Here's how the part is built. I have some questions about the finished solid (model axes, mm). A direction names the side the tool comes from. Coordinates: 2 decimals unless noted, no trailing zeros. Write each loop counter-clockwise with the first axis right and the second up, starting at its lowest first coordinate (ties: lowest second). Pieces come first, ordered by that corner, then holes.
from build123d import *

# Parameters (mm, degrees)
ESQUISSE1_W                     = 50
ESQUISSE1_H                     = 45
MAIN_EXTRUSION_DEPTH            = 20
ESQUISSE5_R                     = 8
GEAR_LINEAR_HOLES_DEPTH         = 21
FIXING_EXTRUSION_DEPTH          = 25
ESQUISSE13_W                    = 50
ESQUISSE13_H                    = 7.2
ROLLINGBALLHORIZONTALHOLE_DEPTH = 11
FRONTHOLE_DEPTH                 = 22
ESQUISSE15_R                    = 1.6
BOTTOMFIXINGHOLE_DEPTH          = 36.1
ESQUISSE12_R                    = 16
REDUCTORMAINHOLE_DEPTH          = 5
REDUCTORFRONTFIXINGHOLE_DEPTH   = 3
ESQUISSE17_R                    = 1.6
MOTORFIXINGHOLE_DEPTH           = 31.1
ESQUISSE19_R                    = 3
ENL_V_MAT_EXTRU_5_DEPTH         = 3
SKETCH2_W                       = 1.5
SKETCH2_H                       = 11
CUTFORMAKERBEAMPROFILE_DEPTH    = 51
CUTFORDISTRIBUTORGRABBER_DEPTH  = 21
SKETCH4_R                       = 1.3
HOLETOBLOCKBEHIND_DEPTH         = 12


with BuildPart() as part:
    # Esquisse1 → Main Extrusion (new body)
    with BuildSketch(Plane.XY):
        Rectangle(ESQUISSE1_W, ESQUISSE1_H)
    extrude(amount=MAIN_EXTRUSION_DEPTH)

    # Esquisse5 → Gear Linear Holes (cut, through all)
    with BuildSketch(Plane.XY.offset(20)):
        with Locations((-7, 2.5)):
            Circle(ESQUISSE5_R)
    extrude(amount=-GEAR_LINEAR_HOLES_DEPTH, mode=Mode.SUBTRACT)

    # Esquisse8 → Fixing Extrusion (add, symmetric)
    with BuildSketch(Plane(origin=(0, 0, 0), x_dir=(0, 0, -1), z_dir=(1, 0, 0))):
        Polygon((-20, -25.5), (-20, -29.05), (-21, -29.05), (-21, -31.95), (-20, -31.95), (-20, -35.5), (0, -35.5), (0, -21.5), (-35.1, -21.5), (-35.1, -35.5), (-30.1, -35.5), (-30.1, -31.95), (-29.1, -31.95), (-29.1, -29.05), (-30.1, -29.05), (-30.1, -25.5), (-26.5, -25.5), (-26.5, -26.5), (-23.6, -26.5), (-23.6, -25.5), align=None)
    extrude(amount=FIXING_EXTRUSION_DEPTH, both=True)

    # Esquisse13 → RollingBallHorizontalHole (cut)
    with BuildSketch(Plane.XY.offset(20)):
        with Locations((0, -14.4)):
            Rectangle(ESQUISSE13_W, ESQUISSE13_H)
    extrude(amount=-ROLLINGBALLHORIZONTALHOLE_DEPTH, mode=Mode.SUBTRACT)

    # Esquisse14 → FrontHole (cut)
    with BuildSketch(Plane.ZY.offset(25)):
        Polygon((0, -23), (20, -23), (20, -18), (35.1, -18), (35.1, -35.5), (0, -35.5), align=None)
    extrude(amount=-FRONTHOLE_DEPTH, mode=Mode.SUBTRACT)

    # Esquisse15 → BottomFixingHole (cut, through all)
    with BuildSketch(Plane.XY.offset(35.1)):
        with Locations((10, -30.5)):
            Circle(ESQUISSE15_R)
    extrude(amount=-BOTTOMFIXINGHOLE_DEPTH, mode=Mode.SUBTRACT)

    # Esquisse12 → ReductorMainHole (cut)
    with BuildSketch(Plane.XY):
        with Locations((-7, 2.5)):
            Circle(ESQUISSE12_R)
    extrude(amount=REDUCTORMAINHOLE_DEPTH, mode=Mode.SUBTRACT)

    # Esquisse16 → ReductorFrontFixingHole (cut)
    with BuildSketch(Plane(origin=(0, 0, 5), x_dir=(-1, 0, 0), z_dir=(0, 0, -1))):
        with BuildLine():
            Line((2.641101056, 11.5), (11.358898944, 11.5))
            ThreePointArc((11.358898944, 11.5), (17, 2.5), (11.358898944, -6.5))
            Line((11.358898944, -6.5), (2.641101056, -6.5))
            ThreePointArc((2.641101056, -6.5), (-3, 2.5), (2.641101056, 11.5))
        make_face()
    extrude(amount=-REDUCTORFRONTFIXINGHOLE_DEPTH, mode=Mode.SUBTRACT)

    # Esquisse17 → MotorFixingHole (cut, through all)
    with BuildSketch(Plane(origin=(0, 0, 5), x_dir=(-1, 0, 0), z_dir=(0, 0, -1))):
        with Locations((-2.192388155, 11.692388155)):
            Circle(ESQUISSE17_R)
        with Locations((16.192388155, 11.692388155)):
            Circle(ESQUISSE17_R)
        with Locations((-2.192388155, -6.692388155)):
            Circle(ESQUISSE17_R)
        with Locations((16.192388155, -6.692388155)):
            Circle(ESQUISSE17_R)
    extrude(amount=-MOTORFIXINGHOLE_DEPTH, mode=Mode.SUBTRACT)

    # Esquisse19 → Enlèv. mat.-Extru.5 (cut)
    with BuildSketch(Plane.XY.offset(20)):
        with Locations((-16.192388155, 11.692388155)):
            Circle(ESQUISSE19_R)
        with Locations((2.192388155, 11.692388155)):
            Circle(ESQUISSE19_R)
        with Locations((-16.192388155, -6.692388155)):
            Circle(ESQUISSE19_R)
        with Locations((2.192388155, -6.692388155)):
            Circle(ESQUISSE19_R)
    extrude(amount=-ENL_V_MAT_EXTRU_5_DEPTH, mode=Mode.SUBTRACT)

    # Sketch2 → CutForMakerBeamProfile (cut, through all)
    with BuildSketch(Plane(origin=(25, 0, 0), x_dir=(0, 0, -1), z_dir=(1, 0, 0))):
        with Locations((-19.25, -14.5)):
            Rectangle(SKETCH2_W, SKETCH2_H)
    extrude(amount=-CUTFORMAKERBEAMPROFILE_DEPTH, mode=Mode.SUBTRACT)

    # Sketch3 → CutForDistributorGrabber (cut, through all)
    with BuildSketch(Plane.XY.offset(20)):
        Polygon((-11, 22.5), (-25, 8.5), (-25, 22.5), align=None)
    extrude(amount=-CUTFORDISTRIBUTORGRABBER_DEPTH, mode=Mode.SUBTRACT)

    # Sketch4 → HoleToBlockBehind (cut)
    with BuildSketch(Plane(origin=(25, 0, 0), x_dir=(0, 0, -1), z_dir=(1, 0, 0))):
        with Locations((-5.05, -30.5)):
            Circle(SKETCH4_R)
        with Locations((-25.05, -30.5)):
            Circle(SKETCH4_R)
        with Locations((-5.05, 17.5)):
            Circle(SKETCH4_R)
        with Locations((-15.05, 17.5)):
            Circle(SKETCH4_R)
    extrude(amount=-HOLETOBLOCKBEHIND_DEPTH, mode=Mode.SUBTRACT)


solid = part.part
1. I want a section at C-C (z = 15.05). List the corners of the cut face in (x, y) for me.
2. Thinking about a two-plate mould opening in Y: for faces 4 (the face through (-22, -9, 19)), 5 (the face through (11, -26.5, 25)), 6 (the face through (25, -6, 14)), which applies, pulls with the +Y half, pulls with the -Y half, needs draft (parallel to the pull), parting line crosses it, or undercut?
3. I want a section at B-B (x = -7). List the corners of the cut face in (y, z) for me, then the cut area to 3 significant figures.
4. For pin 1 Ø20 at (x, y) = (-11, 0.5) entering from -Z; pin 2 Ø0.9 at (x, z) = (-7.5, 6) entering from -Y; pin 3 Ø7 at (x, y) = (-16.19, 11.69) entering from +Z, each with a flat end and sliding along its axis, tell me the tip position at first contact or that it passes through.
5. If I drill on line 1 (Y direction, x = -7, z = 15); line 2 (Y direction, x = 10, z = 12.5); line 3 (Y direction, x = 17.5, z = 12), over which ranges is the centre line in solid material (lowest first)?
6. On a 3-axis mill with a long thin cutter (end or side, diameter ignored), from which of +Z, -Z, +X, -X, +Y, -Y can I reach the whole of each face in a straight line? I mean faces 1 (the face through (11, -34, 20)), 2 (the face through (0, -18, 14)), 3 (the face through (-14.58, 14.22, 18.52)). Say none if no direction works.
7. I want a section at D-D (y = 2.5). List the corners of the cut face in (x, z) for me, then the cut area to 3 significant figures.
8. I want a section at A-A (y = -30.5). List the corners of the cut face in (x, z) for me.
Response values:
1. outline: (-25, -23) - (-3, -23) - (-3, -35.5) - (25, -35.5) - (25, -18) - (-25, -18) - close; (-25, -10.8) - (25, -10.8) - (25, 16.2) - (13, 16.2) - (13, 18.8) - (25, 18.8) - (25, 22.5) - (-11, 22.5) - (-25, 8.5) - close; hole circle Ø3.2 at (-16.19, -6.69); hole circle Ø3.2 at (-16.19, 11.69); hole circle Ø16 at (-7, 2.5); hole circle Ø3.2 at (2.19, -6.69); hole circle Ø3.2 at (2.19, 11.69); hole circle Ø3.2 at (10, -30.5)
2. face 4: undercut
2. face 5: pulls with the -Y half
2. face 6: needs draft
3. outline: (-23, 0) - (-13.5, 0) - (-13.5, 5) - (-6.5, 5) - (-6.5, 8) - (-5.5, 8) - (-5.5, 20) - (-9, 20) - (-9, 18.5) - (-10.8, 18.5) - (-10.8, 9) - (-18, 9) - (-18, 18.5) - (-20, 18.5) - (-20, 20) - (-23, 20) - close; (10.5, 8) - (11.5, 8) - (11.5, 5) - (18.5, 5) - (18.5, 0) - (22.5, 0) - (22.5, 20) - (10.5, 20) - close
3. area: 419 mm2
4. pin 1: stops at z = 5
4. pin 2: stops at y = -23
4. pin 3: stops at z = 20
5. line 1: y = -23 to -18, -10.8 to -5.5, 10.5 to 22.5
5. line 2: y = -35.5 to -32.1, -28.9 to -18, -10.8 to 22.5
5. line 3: y = -35.5 to -18, -10.8 to 22.5
6. face 1: +X, -X, -Y
6. face 2: +Z, +X, -X
6. face 3: +Z
7. outline: (-25, 0) - (-23, 0) - (-23, 5) - (-17, 5) - (-17, 8) - (-15, 8) - (-15, 20) - (-25, 20) - close; (1, 8) - (3, 8) - (3, 5) - (9, 5) - (9, 0) - (25, 0) - (25, 20) - (1, 20) - close
7. area: 588 mm2
8. outline: (-3, 0) - (8.4, 0) - (8.4, 21) - (-3, 21) - close; (-3, 29.1) - (8.4, 29.1) - (8.4, 35.1) - (-3, 35.1) - close; (11.6, 0) - (25, 0) - (25, 3.75) - (13, 3.75) - (13, 6.35) - (25, 6.35) - (25, 21) - (11.6, 21) - close; (11.6, 29.1) - (25, 29.1) - (25, 35.1) - (11.6, 35.1) - close
